Build history of the part. All positions in model axes, mm. A direction names the side the tool comes from. Round coordinates to 2 decimals unless told otherwise and drop trailing zeros. Loops run counter-clockwise (first coordinate to the right, second up) from the corner with the lowest first, then second, coordinate; pieces in that order, holes last. Notation, with made-up numbers: (3, 78.25) - (15, 78.25) arc R8 ccw to (15, 84.25) - close; hole circle Ø2 at (-9, -20.5). An arc over 180 degrees is marked (long way). Put each result on its own line as item: value. Start each with the question number.
from build123d import *

# Parameters (mm, degrees)
F2_ANGLE = 40
F3_COUNT = 4
F4_R     = 6.477
F5_DEPTH = 25.4


with BuildPart() as f1:
    # F0 (on Front) → F1 (revolve)
    with BuildSketch(Plane.XZ):
        with BuildLine():
            Line((0, 25.452), (0, 25.8772801608))
            Line((0, 25.8772801608), (-7.6204296126, 25.8772801608))
            ThreePointArc((-7.6204296126, 25.8772801608), (-13.1374862604, 23.5607943575), (-18.0081613362, 20.0850865393))
            Line((-18.0081613362, 20.0850865393), (-18.0081613362, 19.8241155595))
            Line((-18.0081613362, 19.8241155595), (-15.9627299133, 19.8241155595))
            ThreePointArc((-15.9627299133, 19.8241155595), (-8.46288706, 24.0038298321), (0, 25.452))
        make_face()
        with BuildLine():
            Line((-7.6204296126, 25.8772801608), (-11.9422096565, 25.8772801608))
            ThreePointArc((-11.9422096565, 25.8772801608), (-15.0944548323, 24.1745203327), (-18.0081613362, 22.0897289547))
            Line((-18.0081613362, 22.0897289547), (-18.0081613362, 20.0850865393))
            ThreePointArc((-18.0081613362, 20.0850865393), (-13.1374862604, 23.5607943575), (-7.6204296126, 25.8772801608))
        make_face()
        with BuildLine():
            ThreePointArc((-18.0081613362, 22.0897289547), (-15.0944548323, 24.1745203327), (-11.9422096565, 25.8772801608))
            Line((-11.9422096565, 25.8772801608), (-14.8331613362, 25.8772801608))
            ThreePointArc((-14.8331613362, 25.8772801608), (-17.0782253665, 24.9473441911), (-18.0081613362, 22.7022801608))
            Line((-18.0081613362, 22.7022801608), (-18.0081613362, 22.0897289547))
        make_face()
        with BuildLine():
            ThreePointArc((-18.0081613362, 20.0850865393), (-23.9403569629, 12.4323724401), (-26.7881585713, 3.1779138371))
            Line((-26.7881585713, 3.1779138371), (-25.2528249438, 3.1779138371))
            ThreePointArc((-25.2528249438, 3.1779138371), (-22.2250871425, 12.4036206613), (-15.9627299133, 19.8241155595))
            Line((-15.9627299133, 19.8241155595), (-18.0081613362, 19.8241155595))
            Line((-18.0081613362, 19.8241155595), (-18.0081613362, 20.0850865393))
        make_face()
        with BuildLine():
            ThreePointArc((-26.7881585713, 3.1779138371), (-26.9289986968, 1.5917302503), (-26.976, 0))
            Line((-26.976, 0), (-25.452, 0))
            ThreePointArc((-25.452, 0), (-25.4021574327, 1.5920746731), (-25.2528249438, 3.1779138371))
            Line((-25.2528249438, 3.1779138371), (-26.7881585713, 3.1779138371))
        make_face()
        with BuildLine():
            ThreePointArc((-28.3227948385, 3.1732148584), (-28.4556642243, 1.5890794668), (-28.5, 0))
            Line((-28.5, 0), (-26.976, 0))
            ThreePointArc((-26.976, 0), (-26.9289986968, 1.5917302503), (-26.7881585713, 3.1779138371))
            Line((-26.7881585713, 3.1779138371), (-28.1501204789, 3.1779138371))
            ThreePointArc((-28.1501204789, 3.1779138371), (-28.236489621, 3.176738875), (-28.3227948385, 3.1732148584))
        make_face()
        with BuildLine():
            Line((-31.3251204789, 0), (-28.5, 0))
            ThreePointArc((-28.5, 0), (-28.4556642243, 1.5890794668), (-28.3227948385, 3.1732148584))
            ThreePointArc((-28.3227948385, 3.1732148584), (-30.4554258916, 2.1860748376), (-31.3251204789, 0.0029138371))
            Line((-31.3251204789, 0.0029138371), (-31.3251204789, 0))
        make_face()
    revolve(axis=Axis((0, 0, 14.25), (0, 0, 1)))

    # F0 (on Front) → F2 (revolve)
    with BuildSketch(Plane.XZ):
        with BuildLine():
            ThreePointArc((-18.0081613362, 22.0897289547), (-25.0219503917, 13.6437530979), (-28.3227948385, 3.1732148584))
            ThreePointArc((-28.3227948385, 3.1732148584), (-28.236489621, 3.176738875), (-28.1501204789, 3.1779138371))
            Line((-28.1501204789, 3.1779138371), (-26.7881585713, 3.1779138371))
            ThreePointArc((-26.7881585713, 3.1779138371), (-23.9403569629, 12.4323724401), (-18.0081613362, 20.0850865393))
            Line((-18.0081613362, 20.0850865393), (-18.0081613362, 22.0897289547))
        make_face()
    revolve(axis=Axis((0, 0, 14.25), (0, 0, 1)), revolution_arc=F2_ANGLE)

    # F3: F1 ×4 about axis
    f3_axis = Axis((0, 0, 14.25), (0, 0, 1))


with BuildPart() as f1_1:
    add(f1.part)
    for i in range(1, F3_COUNT):
        add(f1.part.rotate(f3_axis, i * 360 / F3_COUNT))

    # F4 (on face) → F5 (cut)
    with BuildSketch(Plane.XY.offset(25.8772801608)):
        Circle(F4_R)
    extrude(amount=-F5_DEPTH, mode=Mode.SUBTRACT)


solid = f1_1.part
Item 1: Slice it at B-B (z = 23.75). Give the cut face in (x, y), plus the area to 3 significant figures.
Item 2: Drill centre lines: probe 1 along Y at (x, z) = (0, 25.4); probe 2 along X at (y, z) = (-10.5, 6.75); probe 3 along Y at (x, z) = (13.5, 4). Where is each one in solid material? Low to high. Write a range as [from, to].
Item 3: Two-plate mould, pull along Y, no slides. Class faces 6 (the flat face through (11, 25, 3.178)), 7 (the cylindrical face through (-1.404, -6.323, 25.255)), 8 (the flat face through (-24, 0, 13)), 9 (the flat face through (24, 0, 13)): pulls with the +Y half, pulls with the -Y half, needs draft (parallel to the pull), parting line crosses it, or undercut.
Item 4: Slice it at A-A (z = 18.5). Give the cut face in (x, y).
Item 5: Which spindle directions (+Z, -Z, +X, -X, +Y, -Y) get a long thin tool onto all of the face, cutting with end or side? Do faces 1 (the flat face through (15.64, -18.64, 12.68)), 2 (the flat face through (0, -24, 13)), 3 (the flat face through (-15.64, 18.64, 12.68)), 4 (the flat face through (18.64, 15.64, 12.68)), 5 (the flat face through (-18.64, -15.64, 12.68)). Say none if no direction does.
Item 6: Drop flat-ended pins along their axis: pin 1 Ø10 at (y, z) = (6.5, 12.5) entering from +X; pin 2 Ø5.5 at (x, y) = (-21, 15) entering from +Z; pin 3 Ø5 at (y, z) = (23.5, 9) entering from +X; pin 4 Ø11.5 at (x, y) = (0, 0) entering from -Z. Give the stop position or say it passes through.
Computed values:
1. outline: circle Ø35.66 at (0, 0); hole circle Ø18.3 at (0, 0)
1. area: 736 mm^2
2. probe 1: y = [-16.51, -6.48], [6.48, 16.51]
2. probe 2: x = [-25.62, -22.18], [22.18, 23.91]
2. probe 3: y = [-24.78, -21.2], [21.2, 23.01]
3. face 6: needs draft
3. face 7: undercut
3. face 8: pulls with the +Y half
3. face 9: pulls with the -Y half
4. outline: (-21.68, 0) arc R21.68 ccw to (-16.61, -13.94) - (-15.04, -12.62) arc R19.63 ccw to (0, -19.63) - (0, -21.68) arc R21.68 ccw to (13.94, -16.61) - (12.62, -15.04) arc R19.63 ccw to (19.63, 0) - (21.68, 0) arc R21.68 ccw to (16.61, 13.94) - (15.04, 12.62) arc R19.63 ccw to (0, 19.63) - (0, 21.68) arc R21.68 ccw to (-13.94, 16.61) - (-12.62, 15.04) arc R19.63 ccw to (-19.63, 0) - close; hole circle Ø34.96 at (0, 0)
5. face 1: +Z, +X
5. face 2: +Z, -X, -Y
5. face 3: +Z, -X
5. face 4: +Z, +Y
5. face 5: +Z, -Y
6. pin 1: stops at x = 27.01
6. pin 2: stops at z = 14
6. pin 3: stops at x = 14.63
6. pin 4: passes through
